```python
from build123d import *

# Parameters (mm, degrees)
ESQUISSE1_W        = 110
ESQUISSE1_H        = 45
BOSS_EXTRU_1_DEPTH = 40
CONG_1_R           = 10
CONG_2_R           = 10
CONG_3_R           = 10
CONG_4_R           = 10


with BuildPart() as part:
    # Esquisse1 → Boss.-Extru.1 (new body)
    with BuildSketch(Plane.XY):
        with Locations((55, 22.5)):
            Rectangle(ESQUISSE1_W, ESQUISSE1_H)
    extrude(amount=BOSS_EXTRU_1_DEPTH)

    # Congé1
    cong_1_edges = [part.edges().sort_by_distance(p)[0] for p in [
        (0, 22.5, 40),
    ]]
    fillet(cong_1_edges, radius=CONG_1_R)

    # Congé2
    cong_2_edges = [part.edges().sort_by_distance(p)[0] for p in [
        (110, 22.5, 40),
    ]]
    fillet(cong_2_edges, radius=CONG_2_R)

    # Congé3
    cong_3_edges = [part.edges().sort_by_distance(p)[0] for p in [
        (110, 22.5, 0),
    ]]
    fillet(cong_3_edges, radius=CONG_3_R)

    # Congé4
    cong_4_edges = [part.edges().sort_by_distance(p)[0] for p in [
        (0, 22.5, 0),
    ]]
    fillet(cong_4_edges, radius=CONG_4_R)


solid = part.part
```
Here's how the part is built. I have some questions about the finished solid (model axes, mm). Round coordinates to 2 decimals unless told otherwise and drop trailing zeros. Write each loop counter-clockwise with the first axis right and the second up, starting at its lowest first coordinate (ties: lowest second). Pieces come first, ordered by that corner, then holes.
Q1. If we section it at B-B on z = 3: Write out the boundary of the cut face in (x, y), plus the area to 3 significant figures.
Q2. If we section it at A-A on y = 36.5: Write out the boundary of the cut face in (x, z), plus the area to 3 significant figures.
Q3. Please list where these lines run through material, in increasing order: probe 1 along X at (y, z) = (24, 4); probe 2 along X at (y, z) = (4.5, 31); probe 3 along Z at (x, y) = (102, 43.5).
Answer below:
1. outline: (2.86, 0) - (107.14, 0) - (107.14, 45) - (2.86, 45) - close
1. area: 4,690 mm2
2. outline: (0, 10) arc R10 ccw to (10, 0) - (100, 0) arc R10 ccw to (110, 10) - (110, 30) arc R10 ccw to (100, 40) - (10, 40) arc R10 ccw to (0, 30) - close
2. area: 4,310 mm2
3. probe 1: x = 2 to 108
3. probe 2: x = 0.05 to 109.95
3. probe 3: z = 0.2 to 39.8
